```python
from build123d import *

# Parameters (mm, degrees)
F1_DEPTH = 9.525


with BuildPart() as f1:
    # F0 (on Top) → F1 (new body)
    with BuildSketch(Plane.XY):
        with BuildLine():
            Line((0, 2.3), (-387.115837, 2.3))
            ThreePointArc((-387.115837, 2.3), (-395.868834, -6.452997), (-387.115837, -15.205994))
            Line((-387.115837, -15.205994), (-66.557919, -15.205994))
            ThreePointArc((-66.557919, -15.205994), (-63.2144, -15.654019), (-60.106784, -16.966485))
            Line((-60.106784, -16.966485), (-12.860997, -44.827782))
            ThreePointArc((-12.860997, -44.827782), (24.425566, -29.684396), (0, 2.3))
        make_face()
        with BuildLine():
            ThreePointArc((0, 0), (22.206704, -29.078877), (-11.692681, -42.846611))
            Line((-11.692681, -42.846611), (-58.938469, -14.985314))
            ThreePointArc((-58.938469, -14.985314), (-62.608881, -13.435158), (-66.557919, -12.905994))
            Line((-66.557919, -12.905994), (-387.115837, -12.905994))
            ThreePointArc((-387.115837, -12.905994), (-393.568834, -6.452997), (-387.115837, 0))
            Line((-387.115837, 0), (0, 0))
        make_face(mode=Mode.SUBTRACT)
    extrude(amount=F1_DEPTH)


solid = f1.part
```
The listing builds one solid part. Answer for the finished solid, in the listing's coordinates (mm). A direction names the side the tool comes from. Give positions to 0.01 mm unless a question says otherwise; leave off trailing zeros. Order: outer loops, then holes, each group sorted by start corner. A loop starts at its lowest first (then second) coordinate and runs counter-clockwise, first axis right, second up.
1) Determine the mould class of faces 1 (the face through (-395.867, -6.261, 4.696)), 2 (the face through (-36.815, -30.702, 4.696)), 3 (the face through (-225, -12.906, 5)) for opening direction Y: pulls with the +Y half, pulls with the -Y half, needs draft (parallel to the pull), parting line crosses it, or undercut.
Reported:
face 1: parting line crosses it
face 2: pulls with the -Y half
face 3: undercut
2) Consider line 1 along Y through (x, z) = (-232.5, 4); line 2 along X through (y, z) = (-41, 2); line 3 along X through (y, z) = (-38, 6). Determine where each line is inside the solid, lowest interval first.
Reported:
line 1: y = -15.21 to -12.91, 0 to 2.3
line 2: x = -19.35 to -14.82, 14.37 to 17.82
line 3: x = -24.44 to -19.91, 17.48 to 20.41
3) Find section C-C on y = -9. Write down the section's boundary in (x, z) (1 decimal), then the cut area to 3 significant figures.
Reported:
outline: (-395.5, 0) - (-393, 0) - (-393, 9.5) - (-395.5, 9.5) - close; (18.3, 0) - (21.1, 0) - (21.1, 9.5) - (18.3, 9.5) - close
area: 50.2 mm2
4) Find section B-B on x = -194.5. Write down the section's boundary in (y, z) (3 decimals).
Reported:
outline: (-15.206, 0) - (-12.906, 0) - (-12.906, 9.525) - (-15.206, 9.525) - close; (0, 0) - (2.3, 0) - (2.3, 9.525) - (0, 9.525) - close
5) Find section A-A on z = 3.5. Write down the section's boundary in (x, y), then the cut area to 3 significant figures.
Reported:
outline: (-387.12, -15.21) - (-66.56, -15.21) arc R12.7 cw to (-60.11, -16.97) - (-12.86, -44.83) arc R25.32 ccw (long way) to (0, 2.3) - (-387.12, 2.3) arc R8.75 ccw to start; hole (-387.12, -12.91) - (-66.56, -12.91) arc R15 cw to (-58.94, -14.99) - (-11.69, -42.85) arc R23.02 ccw (long way) to (0, 0) - (-387.12, 0) arc R6.45 ccw to start
area: 2,030 mm2
6) For faces 4 (the face through (-171, -14, 0)), 5 (the face through (-62.55, -13.45, 4.7)), 6 (the face through (-229, -15.206, 5)), determine the directions among +Z, -Z, +X, -X, +Y, -Y from which every point of the face is accessible in a straight line to the end or side of a thin tool.
Reported:
face 4: -Z, +X, -X, +Y, -Y
face 5: +Z, -Z
face 6: +Z, -Z, -X, -Y
7) Given P1, Ø5, axis at y = -37.5, z = 4, coming from the +X side; P2, Ø3, axis at x = -264.5, z = 3.5, coming from the -Y side; P3, Ø1, axis at x = -26, y = -35.5, coming from the -Z side, each flat-ended and moving along its own axis, determine where each tip first touches the part or whether it passes through.
Reported:
P1: stops at x = 22.3
P2: stops at y = -15.21
P3: stops at z = 0
